Model file for the job. Use its own axes, mm. Face numbers are marked on the shaded views. Round coordinates to 2 decimals unless told otherwise and drop trailing zeros. Loops run counter-clockwise (first coordinate to the right, second up) from the corner with the lowest first, then second, coordinate; pieces in that order, holes last. Notation, with made-up numbers: M 52.5,12.5 L 109.5,12.5 A3 cw 109.5,16.5 Z; hole C 87,-9.5 d8. An arc over 180 degrees is marked long. Answer in a Markdown table with one row per item.
Autodesk Inventor part; units mm, degrees
ref_plane "YZ Plane" through (0, 0, 0) normal (1, 0, 0) x (0, 1, 0)
ref_plane "XZ Plane" through (0, 0, 0) normal (0, 1, 0) x (-1, 0, 0)
ref_plane "XY Plane" through (0, 0, 0) normal (0, 0, 1) x (1, 0, 0)
sketch "Sketch1" plane through (0, 0, 0) normal (0, 0, 1) x (1, 0, 0)
  line L0 (3.5859, 14.3435) -> (203.5859, 14.3435)
  line L1 (203.5859, 14.3435) -> (203.5859, -185.6565)
  line L2 (203.5859, -185.6565) -> (3.5859, -185.6565)
  line L3 (3.5859, -185.6565) -> (3.5859, 14.3435)
  point P0 (0, 0)
  dimension "d0" = 200
  dimension "d1" = 200
extrude "Extrusion1" add sketch "Sketch1" along normal blind 200
sketch "Sketch2" plane through (0, 0, 200) normal (0, 0, 1) x (1, 0, 0)
  line L0 (203.5859, 14.3435) -> (3.5859, 14.3435)
  line L1 (3.5859, -185.6565) -> (203.5859, -185.6565)
  circle A0 centre (103.5859, -85.6565) radius 45
  point P0 (0, 0)
  dimension "d4" = 90
extrude "Extrusion2" cut sketch "Sketch2" against normal blind 200
thread "Thread1"
sketch "Sketch3" plane through (3.5859, 14.3435, 0) normal (0, 1, 0) x (1, 0, 0)
  line L0 (0, -200) -> (200, -200)
  line L1 (200, 0) -> (200, -200)
  line L2 (0, -200) -> (200, -200)
  line L3 (200, -200) -> (200, 0)
  line L4 (200, 0) -> (0, 0)
  line L5 (0, 0) -> (0, -200)
  point P0 (-3.5859, 0)
extrude "Extrusion3" add sketch "Sketch3" along normal blind 200
fillet "Fillet1" radius 100 2 edges at (103.5859, 214.3435, 0) (103.5859, 214.3435, 200)
sketch "Sketch4" plane through (3.5859, -185.6565, 0) normal (-1, 0, 0) x (0, 0, 1)
  arc A0 (200, 300) -> (0, 300) centre (100, 300) ccw
  circle A1 centre (100, 300) radius 25
  point P0 (0, 185.6565)
  dimension "d12" = 50
hole "Hole1" at (3.5859, 114.3435, 100) direction (1, 0, 0) diameter 100 end through all
properties part number "klocek"
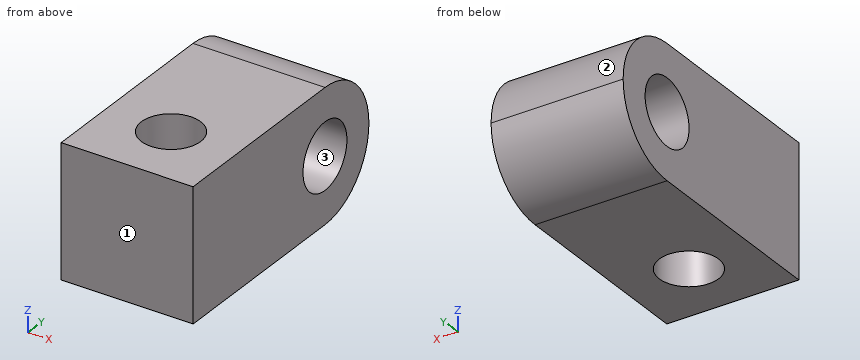
1. Mould opens along Y. For the marked faces 1, 2 and 3 say: +Y half, -Y half, draft (parallel to the pull), parting line (faces both ways), or undercut.
Verdict:
| item | result |
|---|---|
| face 1 | -Y half |
| face 2 | +Y half |
| face 3 | undercut |
2. Saw through at C-C (z = 129). Write the cut outline in (x, y).
Verdict:
| item | result |
|---|---|
| outline | M 3.59,-185.66 L 203.59,-185.66 L 203.59,73.61 L 3.59,73.61 Z; M 3.59,155.07 L 203.59,155.07 L 203.59,210.05 L 3.59,210.05 Z; hole C 103.59,-85.66 d90 |
3. Wall check: probe 1 along Y at (x, z) = (143, 100); probe 2 along Y at (x, z) = (134, 100); probe 3 along Z at (x, y) = (190.5, 116). Give the ranges that are in metal, low to high.
Verdict:
| item | result |
|---|---|
| probe 1 | y = -185.66 to -107.37, -63.94 to 64.34, 164.34 to 214.34 |
| probe 2 | y = -185.66 to -118.82, -52.49 to 64.34, 164.34 to 214.34 |
| probe 3 | z = 0.01 to 50.03, 149.97 to 199.99 |
4. Saw through at B-B (y = 82). Write the cut outline in (x, z), and give its area (3 significant figures).
Verdict:
| item | result |
|---|---|
| outline | M 3.59,0 L 203.59,0 L 203.59,61.87 L 3.59,61.87 Z; M 3.59,138.13 L 203.59,138.13 L 203.59,200 L 3.59,200 Z |
| area | 24,700 mm² |
5. Saw through at A-A (x = 69). State how many separate pieces and enclosed holes the cut face has, and give its area (3 significant figures).
Verdict:
| item | result |
|---|---|
| separate pieces | 2 |
| enclosed holes | 1 |
| area | 56,300 mm² |
6. Pin check, flat tips, straight feed: pin 1 (3 mm diameter, centred on x = 91, z = 94, fed in from +Y); pin 2 (1.5 mm diameter, centred on x = 59, z = 115.5, fed in from +Y). Stop position of each tip, or through.
Verdict:
| item | result |
|---|---|
| pin 1 | stops at y = 214.24 |
| pin 2 | stops at y = 213.25 |
